from build123d import *

# Parameters (mm, degrees)
CROQUIS1_R              = 2.75
CROQUIS1_R_2            = 8
SALIENTE_EXTRUIR1_DEPTH = 4


with BuildPart() as part:
    # Croquis1 → Saliente-Extruir1 (new body)
    with BuildSketch(Plane(origin=(0, 0, 0), x_dir=(1, 0, 0), z_dir=(0, 1, 0))):
        with BuildLine():
            Line((-19.683050508, 22.941797025), (-19.683050508, -35.249327106))
            ThreePointArc((-19.683050508, -35.249327106), (-18.218584414, -38.784861012), (-14.683050508, -40.249327106))
            Line((-14.683050508, -40.249327106), (-4.549566926, -40.249327106))
            ThreePointArc((-4.549566926, -40.249327106), (-1.01403302, -38.784861012), (0.450433074, -35.249327106))
            Line((0.450433074, -35.249327106), (0.450433074, -25.249327106))
            ThreePointArc((0.450433074, -25.249327106), (1.914899168, -21.7137932), (5.450433074, -20.249327106))
            Line((5.450433074, -20.249327106), (15.316949492, -20.249327106))
            ThreePointArc((15.316949492, -20.249327106), (18.852483398, -18.784861012), (20.316949492, -15.249327106))
            Line((20.316949492, -15.249327106), (20.316949492, -5.249327106))
            ThreePointArc((20.316949492, -5.249327106), (18.852483398, -1.7137932), (15.316949492, -0.249327106))
            Line((15.316949492, -0.249327106), (13.97720353, -0.249327106))
            ThreePointArc((13.97720353, -0.249327106), (11.023751057, 0.716181787), (9.210932436, 3.239825498))
            Line((9.210932436, 3.239825498), (1.302567045, 28.188350052))
            ThreePointArc((1.302567045, 28.188350052), (-11.475083798, 39.388167744), (-19.998351013, 24.689249641))
            ThreePointArc((-19.998351013, 24.689249641), (-19.762506967, 23.82963218), (-19.683050508, 22.941797025))
        make_face()
        with Locations(Location((10.316949492, -10.460860181, 0), (0, 0, 270))):
            Circle(CROQUIS1_R, mode=Mode.SUBTRACT)
        with Locations(Location((-9.683050508, -10.460860181, 0), (0, 0, 270))):
            Circle(CROQUIS1_R, mode=Mode.SUBTRACT)
        with Locations(Location((-9.683050508, -30.460860181, 0), (0, 0, 270))):
            Circle(CROQUIS1_R, mode=Mode.SUBTRACT)
        with Locations(Location((-9.692012125, 28.533645396, 0), (0, 0, 270))):
            Circle(CROQUIS1_R_2, mode=Mode.SUBTRACT)
    extrude(amount=SALIENTE_EXTRUIR1_DEPTH)


solid = part.part
Design review of the part built by this model. Coordinates are the model's own, in mm. A direction names the side the tool comes from. Give positions to 0.01 mm unless a question says otherwise; leave off trailing zeros. Order: outer loops, then holes, each group sorted by start corner. A loop starts at its lowest first (then second) coordinate and runs counter-clockwise, first axis right, second up.
1. Add section A-A, the plane x = -8. State the section outline as (y, z) points.
Solution:
outline: (0, -39.4) - (4, -39.4) - (4, -36.35) - (0, -36.35) - close; (0, -20.71) - (4, -20.71) - (4, 8.29) - (0, 8.29) - close; (0, 12.64) - (4, 12.64) - (4, 28.29) - (0, 28.29) - close; (0, 32.64) - (4, 32.64) - (4, 40.25) - (0, 40.25) - close
2. To check wall thickness, follow L1, parallel to Z at x = -9.5, y = 3; L2, parallel to Z at x = -11, y = 0.55; L3, parallel to X at y = 1.4, z = -27. State the ranges of each line that lie inside material, in increasing order.
Solution:
L1: z = -39.53 to -36.53, -20.54 to 7.72, 13.2 to 27.72, 33.2 to 40.25
L2: z = -39.46 to -36.43, -20.64 to 8.05, 12.88 to 28.05, 32.88 to 40.25
L3: x = -20.58 to -17.54, -1.84 to 1.68
3. Add section C-C, the plane y = 1.95. State the section outline as (x, z) points.
Solution:
outline: (-20, -24.69) arc R11 ccw (long way) to (1.3, -28.19) - (9.21, -3.24) arc R5 cw to (13.98, 0.25) - (15.32, 0.25) arc R5 ccw to (20.32, 5.25) - (20.32, 15.25) arc R5 ccw to (15.32, 20.25) - (5.45, 20.25) arc R5 cw to (0.45, 25.25) - (0.45, 35.25) arc R5 ccw to (-4.55, 40.25) - (-14.68, 40.25) arc R5 ccw to (-19.68, 35.25) - (-19.68, -22.94) arc R5 cw to start; hole circle Ø16 at (-9.69, -28.53); hole circle Ø5.5 at (-9.68, 10.46); hole circle Ø5.5 at (-9.68, 30.46); hole circle Ø5.5 at (10.32, 10.46)
4. Add section D-D, the plane x = 4. State the section outline as (y, z) points, then the cut area to 3 significant figures.
Solution:
outline: (0, -19.68) - (4, -19.68) - (4, 20.46) - (0, 20.46) - close
area: 161 mm2
5. Add section B-B, the plane z = 34.5. State the section outline as (x, y) points, then the cut area to 3 significant figures.
Solution:
outline: (-19.68, 0) - (0.45, 0) - (0.45, 4) - (-19.68, 4) - close
area: 80.5 mm2
6. Mouldability with a two-part tool opening along Z and no side actions: class faces 3 (the cylindrical face through (11.06, 1.97, -0.69)), 4 (the flat face through (10, 2, 20.249)), 5 (the cylindrical face through (-9.34, 1.972, -36.526)), 6 (the flat face through (20.317, 2, 10)) as +Z half, -Z half, draft (parallel to the pull), parting line (faces both ways), or undercut.
Solution:
face 3: -Z half
face 4: +Z half
face 5: undercut
face 6: draft
7. Tool access review of faces 1 (the flat face through (-5, 4, 9)), 2 (the flat face through (0.45, 2, 30)): name each direction out of +Z, -Z, +X, -X, +Y, -Y from which nothing blocks a thin tool from reaching the whole face with its end or side.
Solution:
face 1: +Z, -Z, +X, -X, +Y
face 2: +Z, +X, +Y, -Y
8. For pin 1 Ø1.1 at (x, y) = (14.5, 1) entering from -Z; pin 2 Ø1.5 at (x, y) = (9.5, 3) entering from +Z; pin 3 Ø2 at (y, z) = (2, 7.5) entering from -X, all flat-tipped, find the tip position at first contact; note any pin that passes through.
Solution:
pin 1: stops at z = 0.25
pin 2: stops at z = 20.25
pin 3: stops at x = -19.68
